Design review of the part built by this model. Coordinates are the model's own, in mm. A direction names the side the tool comes from. Coordinates: 2 decimals unless noted, no trailing zeros. Order: outer loops, then holes, each group sorted by start corner. A loop starts at its lowest first (then second) coordinate and runs counter-clockwise, first axis right, second up. Notation, with made-up numbers: M 22,-20 L 69,-20 A13 ccw 69,2 Z; hole C -23,36 d3. An arc over 180 degrees is marked long. Answer as a JSON object with one key per item and string values.
Autodesk Inventor part; units mm, degrees
ref_plane "YZ Plane" through (0, 0, 0) normal (1, 0, 0) x (0, 1, 0)
ref_plane "XZ Plane" through (0, 0, 0) normal (0, 1, 0) x (-1, 0, 0)
ref_plane "XY Plane" through (0, 0, 0) normal (0, 0, 1) x (1, 0, 0)
sketch "스케치1" plane through (0, 0, 0) normal (0, 1, 0) x (-1, 0, 0)
  line L0 (0, 0) -> (-315, 0)
  line L1 (-315, 0) -> (-315, -950)
  line L2 (-315, -950) -> (0, -950)
  line L3 (0, -950) -> (0, 0)
  line L4 (-315, -645) -> (-315, -475)
  line L5 (-315, -475) -> (-535, -475)
  line L6 (-535, -475) -> (-535, -645)
  line L7 (-535, -645) -> (-315, -645)
  line L8 (-315, -645) -> (-315, -475)
  line L9 (-315, -475) -> (-535, -475)
  line L10 (-315, -305) -> (-315, -475)
  line L11 (-315, -475) -> (-535, -475)
  line L12 (-535, -475) -> (-535, -305)
  line L13 (-535, -305) -> (-315, -305)
  line L14 (-315, -305) -> (-315, -475)
  line L15 (0, -305) -> (0, 0)
  line L16 (0, -645) -> (0, -950)
  line L17 (0, 0) -> (175, 0)
  line L18 (175, 0) -> (175, -950)
  line L19 (175, -950) -> (0, -950)
  line L20 (0, -950) -> (0, 0)
  line L21 (175, 0) -> (145, 0)
  line L22 (145, 0) -> (145, -950)
  line L23 (145, -950) -> (175, -950)
  line L24 (175, -950) -> (175, 0)
  line L25 (175, -475) -> (145, -475)
  line L26 (145, -475) -> (145, -645)
  line L27 (145, -645) -> (175, -645)
  line L28 (175, -645) -> (175, -475)
  line L29 (175, -475) -> (145, -475)
  line L30 (145, -475) -> (145, -305)
  line L31 (145, -305) -> (175, -305)
  line L32 (175, -305) -> (175, -475)
  line L33 (145, -645) -> (-315, -645)
  line L34 (-315, -645) -> (-315, -685)
  line L35 (-315, -685) -> (145, -685)
  line L36 (145, -685) -> (145, -645)
  line L37 (145, -305) -> (-315, -305)
  line L38 (-315, -305) -> (-315, -265)
  line L39 (-315, -265) -> (145, -265)
  line L40 (145, -265) -> (145, -305)
  line L41 (0, 0) -> (145, -265)
  line L42 (145, -685) -> (0, -950)
  dimension "d0" = 315
  dimension "d1" = 950
  dimension "d3" = 220
  dimension "d4" = 170
  dimension "d5" = 220
  dimension "d6" = 170
  dimension "d7" = 175
  dimension "d8" = 30
  dimension "d9" = 460
  dimension "d10" = 40
  dimension "d11" = 460
  dimension "d12" = 40
extrude "돌출1" add sketch "스케치1" along normal blind 20 contours L3 L39 L1 L0 | L41 L39 L3 | L39 L22 L37 L3 | L3 L37 L1 L39 | L37 L22 L33 L3 | L3 L33 L1 L37 | L31 L18 L25 L22 | L1 L5 L12 L13 | L33 L22 L35 L3 | L3 L35 L1 L33 | L25 L18 L27 L22 | L1 L7 L6 L5 | L35 L42 L3 | L3 L2 L1 L35
properties part number "cover" material "청동, 주조"
1) Add section B-B (x = 456.5). State the section outline as (y, z) points, and give its area (3 significant figures).
Taken from the geometry:
{"outline": "M 0,-645 L 20,-645 L 20,-305 L 0,-305 Z", "area": "6,800 mm2"}
2) Insertion check: pin 1 Ø12 at (y, z) = (5.5, -254.5) entering from -X; pin 2 Ø10 at (y, z) = (5.5, -666) entering from -X; pin 3 Ø2 at (x, y) = (-92, 6) entering from +Z. Each pin has a flat end and moves straight along its axis. Give the tip position at first contact, or say it passes through.
Taken from the geometry:
{"pin 1": "stops at x = -142.54", "pin 2": "stops at x = -145", "pin 3": "stops at z = -166.31"}
3) Add section C-C (z = -850). State the section outline as (x, y) points, and give its area (3 significant figures).
Taken from the geometry:
{"outline": "M -54.72,0 L 315,0 L 315,20 L -54.72,20 Z", "area": "7,390 mm2"}
4) Add section A-A (y = 14.25). State the section outline as (x, z) points, and give its area (3 significant figures).
Taken from the geometry:
{"outline": "M -175,-645 L -145,-645 L -145,-685 L 0,-950 L 315,-950 L 315,-645 L 535,-645 L 535,-305 L 315,-305 L 315,0 L 0,0 L -145,-265 L -145,-305 L -175,-305 Z", "area": "484,000 mm2"}
5) Tool access review of faces 1 (the flat face through (315, 10, -795)), 2 (the flat face through (-145, 10, -665)), 3 (the flat face through (-145, 10, -285)), 4 (the flat face through (427, 10, -305)): name each direction out of +Z, -Z, +X, -X, +Y, -Y from which nothing blocks a thin tool from reaching the whole face with its end or side.
Taken from the geometry:
{"face 1": "-Z, +X, +Y, -Y", "face 2": "-Z, -X, +Y, -Y", "face 3": "+Z, -X, +Y, -Y", "face 4": "+Z, +X, +Y, -Y"}
6) To check wall thickness, follow L1, parallel to Z at x = 428.5, y = 18; L2, parallel to X at y = 3.75, z = -292; L3, parallel to X at y = 9.25, z = -66.5. State the ranges of each line that lie inside material, in increasing order.
Taken from the geometry:
{"L1": "z = -645 to -305", "L2": "x = -145 to 315", "L3": "x = -36.39 to 315"}
